from build123d import *

# Parameters (mm, degrees)
SKETCH001_W     = 103.5
SKETCH001_H     = 33
PAD_DEPTH       = 1.5
SKETCH002_W     = 103.5
SKETCH002_H     = 33
SKETCH002_W_2   = 100.5
SKETCH002_H_2   = 30
PAD001_DEPTH    = 14
SKETCH003_R     = 1.15
SKETCH003_R_2   = 2
SKETCH003_R_3   = 0.75
PAD002_DEPTH    = 10
SKETCH004_W     = 4.4
SKETCH004_H     = 4.4
PAD003_DEPTH    = 8.5
FILLET_R        = 1.15
SKETCH005_R     = 2
POCKET_DEPTH    = 3.5
SKETCH006_W     = 9.999999
SKETCH006_H     = 7.5
POCKET001_DEPTH = 16.6
FILLET001_R     = 1.5
FILLET002_R     = 1.5
FILLET003_R     = 3


with BuildPart() as part:
    # Sketch001 → Pad (new body)
    with BuildSketch(Plane.XY):
        Rectangle(SKETCH001_W, SKETCH001_H)
    extrude(amount=-PAD_DEPTH)

    # Sketch002 (on Face5 of Pad) → Pad001 (join)
    with BuildSketch(Plane.XY):
        Rectangle(SKETCH002_W, SKETCH002_H)
        Rectangle(SKETCH002_W_2, SKETCH002_H_2, mode=Mode.SUBTRACT)
    extrude(amount=PAD001_DEPTH)

    # Sketch003 (on Face15 of Pad001) → Pad002 (join)
    with BuildSketch(Plane.XY):
        with Locations((4, -11.75)):
            Circle(SKETCH003_R)
        with Locations((-47, -11.75)):
            Circle(SKETCH003_R)
        with Locations((-47, 11.75)):
            Circle(SKETCH003_R)
        with Locations((4, 11.75)):
            Circle(SKETCH003_R)
        with Locations((17.25, 10)):
            Circle(SKETCH003_R_2)
        with Locations((17.25, 10)):
            Circle(SKETCH003_R_3, mode=Mode.SUBTRACT)
        with Locations((17.25, -10)):
            Circle(SKETCH003_R_2)
        with Locations((17.25, -10)):
            Circle(SKETCH003_R_3, mode=Mode.SUBTRACT)
        with Locations((47.25, 0)):
            Circle(SKETCH003_R_2)
        with Locations((47.25, 0)):
            Circle(SKETCH003_R_3, mode=Mode.SUBTRACT)
    extrude(amount=PAD002_DEPTH)

    # Sketch004 (on Face15 of Pad002) → Pad003 (join)
    with BuildSketch(Plane.XY):
        with Locations((-48.05, 12.8)):
            Rectangle(SKETCH004_W, SKETCH004_H)
        with Locations((-48.05, -12.8)):
            Rectangle(SKETCH004_W, SKETCH004_H)
        with Locations((5.05, 12.8)):
            Rectangle(SKETCH004_W, SKETCH004_H)
        with Locations((5.05, -12.8)):
            Rectangle(SKETCH004_W, SKETCH004_H)
    extrude(amount=PAD003_DEPTH)

    # Fillet
    fillet_edges = [part.edges().sort_by_distance(p)[0] for p in [
        (45.25, 0, 0),
        (15.25, 10, 0),
        (15.25, -10, 0),
        (2.85, 13.375, 0),
        (2.85, 11.175, 0),
        (2.85, -11.175, 0),
        (2.85, -13.375, 0),
        (7.25, 12.8, 0),
        (7.25, -12.8, 0),
    ]]
    fillet(fillet_edges, radius=FILLET_R)

    # Sketch005 (on Face62 of Fillet) → Pocket (cut)
    with BuildSketch(Plane.XY.offset(10)):
        with Locations((17.25, 10)):
            Circle(SKETCH005_R)
        with Locations((17.25, -10)):
            Circle(SKETCH005_R)
        with Locations((47.25, 0)):
            Circle(SKETCH005_R)
    extrude(amount=-POCKET_DEPTH, mode=Mode.SUBTRACT)

    # Sketch006 → Pocket001 (cut, symmetric)
    with BuildSketch(Plane.XZ):
        with Locations((33.916666, 10.25)):
            Rectangle(SKETCH006_W, SKETCH006_H)
    extrude(amount=POCKET001_DEPTH, both=True, mode=Mode.SUBTRACT)

    # Fillet001
    fillet001_edges = [part.edges().sort_by_distance(p)[0] for p in [
        (38.916666, -15.75, 6.5),
        (38.916666, 15.75, 6.5),
        (28.916667, -15.75, 6.5),
        (28.916667, 15.75, 6.5),
    ]]
    fillet(fillet001_edges, radius=FILLET001_R)

    # Fillet002
    fillet002_edges = [part.edges().sort_by_distance(p)[0] for p in [
        (50.25, 15, 7),
        (50.25, -15, 7),
        (-50.25, 15, 11.25),
        (-50.25, -15, 11.25),
    ]]
    fillet(fillet002_edges, radius=FILLET002_R)

    # Fillet003
    fillet003_edges = [part.edges().sort_by_distance(p)[0] for p in [
        (-51.75, -16.5, 7),
        (51.75, -16.5, 7),
        (51.75, 16.5, 7),
        (-51.75, 16.5, 7),
    ]]
    fillet(fillet003_edges, radius=FILLET003_R)


solid = part.part
Source: CAD feature listing. Evaluate the final solid. Frame: model axes, mm. A direction names the side the tool comes from. Round coordinates to 2 decimals unless told otherwise and drop trailing zeros. Loops run counter-clockwise (first coordinate to the right, second up) from the corner with the lowest first, then second, coordinate; pieces in that order, holes last. Notation, with made-up numbers: (-16.5, -8.5) - (8.5, -8.5) arc R27 ccw to (8.5, 24.5) - close; hole circle Ø5 at (85.25, -26.5). An arc over 180 degrees is marked (long way). Write item = value, one per line. Start each with the question number.
Item 1: Section query B-B on z = 12.5. Output: boundary loops of the cut face in (x, y).
Item 2: First-contact query: pin 1 Ø0.8 at (y, z) = (-16, 11.5) entering from +X; pin 2 Ø1.5 at (x, y) = (-6, 4.5) entering from +Z; pin 3 Ø1.2 at (x, y) = (17, 10) entering from +Z. Flat tips, straight axial feed; report the tip coordinate or a pass-through.
Item 3: Reachability of faces 1 (the face through (-1, 0, -1.5)), 2 (the face through (7.25, -13, 5)) from +Z, -Z, +X, -X, +Y, -Y: full face, straight path, thin tool, end or side. Return the list, or none.
Item 4: Section query A-A on z = 5. Count the separate pieces of the cut face and the enclosed holes in it, plus the area to 3 significant figures.
Item 5: Mould query, pull axis X, two halves, no side actions, for faces 3 (the face through (-45.85, 13, 4)), 4 (the face through (-24, -16, 14)), 5 (the face through (51.75, 0, 6)), 6 (the face through (-50.85, 15.64, 6.14)). Classes: released by +X, released by -X, zero draft, split by the parting line, or undercut.
Item 6: Material intervals for line 1 (Y direction, x = 17.25, z = 3.5); line 2 (X direction, y = 0, z = 4.5); line 3 (X direction, y = 12, z = 7.5), sorted ascending.
Results list:
q1.outline = (-51.75, -13.5) arc R3 ccw to (-48.75, -16.5) - (28.92, -16.5) - (28.92, -15) - (-48.75, -15) arc R1.5 cw to (-50.25, -13.5) - (-50.25, 13.5) arc R1.5 cw to (-48.75, 15) - (28.92, 15) - (28.92, 16.5) - (-48.75, 16.5) arc R3 ccw to (-51.75, 13.5) - close; (38.92, -16.5) - (48.75, -16.5) arc R3 ccw to (51.75, -13.5) - (51.75, 13.5) arc R3 ccw to (48.75, 16.5) - (38.92, 16.5) - (38.92, 15) - (48.75, 15) arc R1.5 cw to (50.25, 13.5) - (50.25, -13.5) arc R1.5 cw to (48.75, -15) - (38.92, -15) - close
q2.pin_1 = 50.89
q2.pin_2 = 0
q2.pin_3 = 6.5
q3.face_1 = -Z, +X, -X, +Y, -Y
q3.face_2 = +Z
q4.separate_pieces = 4
q4.enclosed_holes = 4
q4.area = 504 mm²
q5.face_3 = undercut
q5.face_4 = zero draft
q5.face_5 = released by +X
q5.face_6 = released by -X
q6.line_1 = -16.5 to -15, -12 to -10.75, -9.25 to -8, 8 to 9.25, 10.75 to 12, 15 to 16.5
q6.line_2 = -51.75 to -50.25, 45.25 to 46.5, 48 to 49.25, 50.25 to 51.75
q6.line_3 = -51.75 to -45.85, 2.85 to 7.25, 50.25 to 51.75
